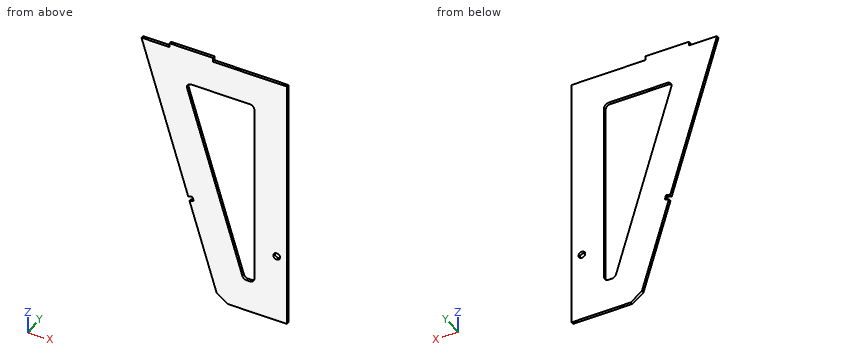
```python
from build123d import *

# Parameters (mm, degrees)
BOSS_EXTRUDE1_DEPTH = 3.175
SKETCH4_W           = 50.8
SKETCH4_H           = 3.175
BOSS_EXTRUDE2_DEPTH = 4.7625
SKETCH6_W           = 300.355
SKETCH6_H           = 3.175
BOSS_EXTRUDE3_DEPTH = 53.8189678
SKETCH7_R           = 3.96875
CUT_EXTRUDE3_DEPTH  = 322.952646539
CUT_EXTRUDE4_DEPTH  = 322.952646539
FILLET1_R           = 5.08
CUT_EXTRUDE5_DEPTH  = 322.952646539


with BuildPart() as part:
    # Sketch2 → Boss-Extrude1 (new body)
    with BuildSketch(Plane(origin=(0, 0, 0), x_dir=(1, 0, 0), z_dir=(0, 1, 0))):
        Polygon((0, 0), (-115.889171037, 0), (-25.4, 300.355), (0, 300.355), align=None)
    extrude(amount=BOSS_EXTRUDE1_DEPTH)

    # Sketch4 → Boss-Extrude2 (add)
    with BuildSketch(Plane.XY):
        with Locations((-57.944585519, 1.5875)):
            Rectangle(SKETCH4_W, SKETCH4_H)
    extrude(amount=BOSS_EXTRUDE2_DEPTH)

    # Sketch6 → Boss-Extrude3 (add)
    with BuildSketch(Plane(origin=(0, 0, 0), x_dir=(0, 0, -1), z_dir=(1, 0, 0))):
        with Locations((150.1775, 1.5875)):
            Rectangle(SKETCH6_W, SKETCH6_H)
    extrude(amount=BOSS_EXTRUDE3_DEPTH)

    # Sketch7 → Cut-Extrude3 (cut, through all)
    with BuildSketch(Plane(origin=(0, 3.175, 0), x_dir=(1, 0, 0), z_dir=(0, 1, 0))):
        with Locations(Location((41.7539678, 219.202, 0), (0, 0, 270))):
            Circle(SKETCH7_R)
        Polygon((-28.330823353, 290.626902834), (-15.24, 300.355), (-25.4, 300.355), align=None)
    extrude(amount=-CUT_EXTRUDE3_DEPTH, mode=Mode.SUBTRACT)

    # Sketch8 → Cut-Extrude4 (cut, through all)
    with BuildSketch(Plane(origin=(0, 3.175, 0), x_dir=(1, 0, 0), z_dir=(0, 1, 0))):
        Polygon((-64.619085916, 38.1), (15.7189678, 38.1), (15.7189678, 262.255), (2.91300156, 262.255), align=None)
    extrude(amount=-CUT_EXTRUDE4_DEPTH, mode=Mode.SUBTRACT)

    # Fillet1
    fillet1_edges = [part.edges().sort_by_distance(p)[0] for p in [
        (-64.619085916, 1.5875, -38.1),
        (2.91300156, 1.5875, -262.255),
        (15.7189678, 1.5875, -262.255),
        (15.7189678, 1.5875, -38.1),
    ]]
    fillet(fillet1_edges, radius=FILLET1_R)

    # Sketch9 → Cut-Extrude5 (cut, through all)
    with BuildSketch(Plane(origin=(0, 3.175, 0), x_dir=(1, 0, 0), z_dir=(0, 1, 0))):
        Polygon((-59.837174403, 186.0498583), (-54.97312582, 184.584446623), (-56.438537497, 179.72039804), (-61.30258608, 181.185809717), align=None)
    extrude(amount=-CUT_EXTRUDE5_DEPTH, mode=Mode.SUBTRACT)


solid = part.part
```
Build history of the part. All positions in model axes, mm. Give positions to 0.01 mm unless a question says otherwise; leave off trailing zeros. Loops run counter-clockwise (first coordinate to the right, second up) from the corner with the lowest first, then second, coordinate; pieces in that order, holes last.
1) Band-saw the part on A-A on z = -176. List the corners of the cut face in (x, y) (3 decimals).
Values follow:
outline: (-62.865, 0) - (-23.073, 0) - (-23.073, 3.175) - (-62.865, 3.175) - close; (15.719, 0) - (53.819, 0) - (53.819, 3.175) - (15.719, 3.175) - close
2) Band-saw the part on C-C on y = 1.3. List the corners of the cut face in (x, z) (1 decimal), then the cut area to 3 significant figures.
Values follow:
outline: (-115.9, 0) - (-61.3, -181.2) - (-56.4, -179.7) - (-55, -184.6) - (-59.8, -186) - (-28.3, -290.6) - (-15.2, -300.4) - (53.8, -300.4) - (53.8, 0) - (-32.5, 0) - (-32.5, 4.8) - (-83.3, 4.8) - (-83.3, 0) - close; hole (-62.6, -44.6) - (1.8, -258.6) arc R5.1 ccw to (6.7, -262.3) - (10.6, -262.3) arc R5.1 ccw to (15.7, -257.2) - (15.7, -43.2) arc R5.1 ccw to (10.6, -38.1) - (-57.8, -38.1) arc R5.1 ccw to start; hole circle Ø7.9 at (41.8, -219.2)
area: 27,100 mm2
3) Probe line 1 along Z through (x, y) = (7, 2) (3 decimals); line 2 along Z through (x, y) = (20, 1.45) (3 decimals); line 3 along Z through (x, y) = (40, 1.1) (3 decimals). List the from-to ranges inside material, lowest first.
Values follow:
line 1: z = -300.355 to -262.255, -38.1 to 0
line 2: z = -300.355 to 0
line 3: z = -300.355 to -222.762, -215.642 to 0
4) Band-saw the part on D-D on z = -13.5. List the corners of the cut face in (x, y) (3 decimals).
Values follow:
outline: (-111.822, 0) - (53.819, 0) - (53.819, 3.175) - (-111.822, 3.175) - close
5) Drop flat-ended pins along their axis: P1, Ø1.6, axis at y = 1.5, z = 2.5, coming from the +X side; P2, Ø1, axis at x = 29.5, y = 1.5, coming from the +Z side; P3, Ø1, axis at y = 2.5, z = 1.5, coming from the -X side; P4, Ø10, axis at x = -91, z = -117, coming from the +Y side. Give the stop position or say it passes through.
Values follow:
P1: stops at x = -32.54
P2: stops at z = 0
P3: stops at x = -83.34
P4: passes through
6) Band-saw the part on B-B on x = -3. List the corners of the cut face in (y, z) (3 decimals), then the cut area to 3 significant figures.
Values follow:
outline: (0, -300.355) - (3.175, -300.355) - (3.175, -242.628) - (0, -242.628) - close; (0, -38.1) - (3.175, -38.1) - (3.175, 0) - (0, 0) - close
area: 304 mm2
